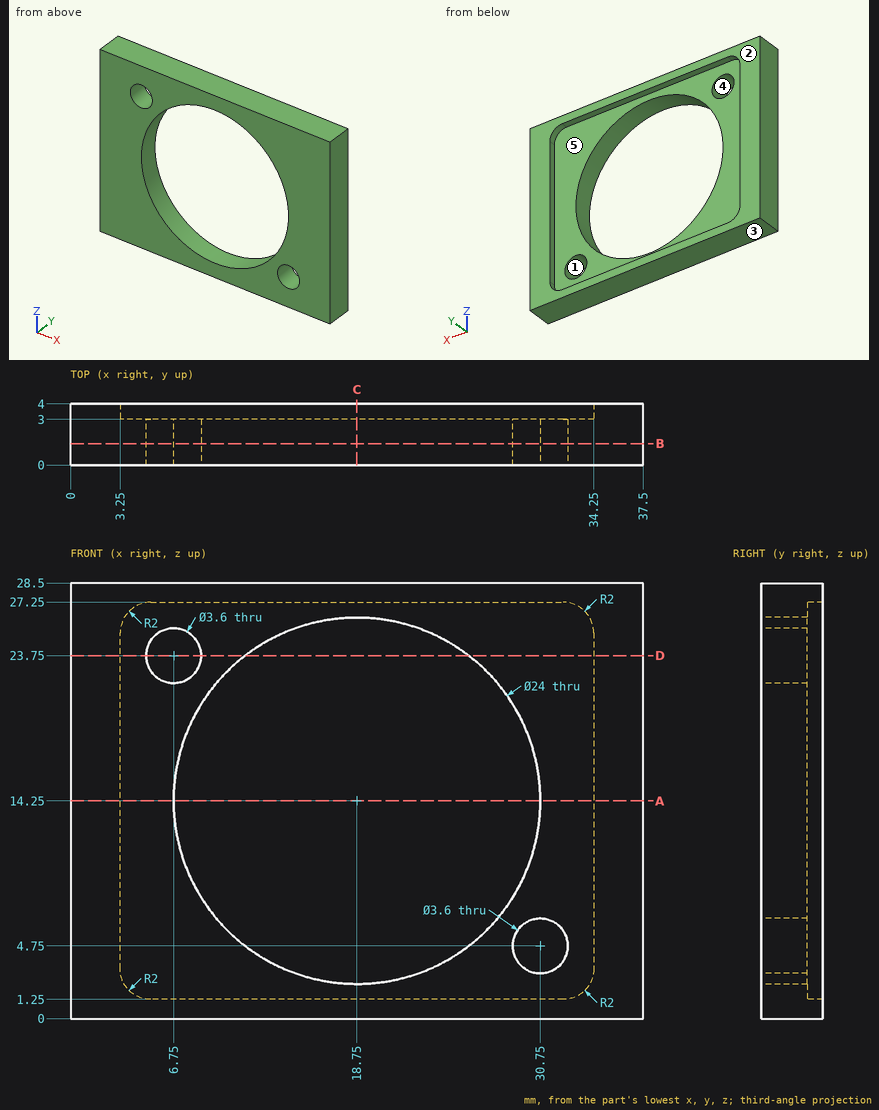
Check sheet for the drawn part. Datum: minimum x, y, z corner. Units: mm. A direction names the side the tool comes from. Give positions to 0.01 mm unless a question says otherwise; leave off trailing zeros. Loops run counter-clockwise (first coordinate to the right, second up) from the corner with the lowest first, then second, coordinate; pieces in that order, holes last. Notation, with made-up numbers: (17, 17) - (60, 17) arc R19 cw to (60, 46) - close; hole circle Ø3 at (-6, 11). An arc over 180 degrees is marked (long way). Write each question's results on one line, items separated by ' | '.
1) Mould release check, pull along Z, two halves, no side actions. Record for the marked faces 1, 2 and 3: pulls with the +Z half, pulls with the -Z half, needs draft (parallel to the pull), parting line crosses it, or undercut.
Solution:
face 1: undercut | face 2: needs draft | face 3: pulls with the -Z half
2) Depth check by flat-ended pin: P1, Ø4, axis at x = 6.75, z = 23.75, coming from the +Y side. Enter the tip coordinate at first touch or a pass-through.
Solution:
P1: y = 3
3) Sectioned sample at A-A on z = 14.25. Record the boundary of the cut face in (x, y), plus the area to 3 significant figures.
Solution:
outline: (0, 0) - (6.75, 0) - (6.75, 3) - (3.25, 3) - (3.25, 4) - (0, 4) - close; (30.75, 0) - (37.5, 0) - (37.5, 4) - (34.25, 4) - (34.25, 3) - (30.75, 3) - close | area: 47.0 mm2
4) Sectioned sample at B-B on y = 1.4. Record the boundary of the cut face in (x, z).
Solution:
outline: (0, 0) - (37.5, 0) - (37.5, 28.5) - (0, 28.5) - close; hole circle Ø3.6 at (6.75, 23.75); hole circle Ø24 at (18.75, 14.25); hole circle Ø3.6 at (30.75, 4.75)
5) Material ranges on L1, parallel to X at y = 1.45, z = 14.25; L2, parallel to Z at x = 27, y = 3.5; L3, parallel to X at y = 3.8, z = 17.75, recorded low to high. Write a range as from..to.
Solution:
L1: 0..6.75, 30.75..37.5 | L2: 0..1.25, 27.25..28.5 | L3: 0..3.25, 34.25..37.5
6) Sectioned sample at C-C on x = 18.75. Record the boundary of the cut face in (y, z), plus the area to 3 significant figures.
Solution:
outline: (0, 0) - (4, 0) - (4, 1.25) - (3, 1.25) - (3, 2.25) - (0, 2.25) - close; (0, 26.25) - (3, 26.25) - (3, 27.25) - (4, 27.25) - (4, 28.5) - (0, 28.5) - close | area: 16.0 mm2
7) Sectioned sample at D-D on z = 23.75. Record the boundary of the cut face in (x, y).
Solution:
outline: (0, 0) - (4.95, 0) - (4.95, 3) - (3.25, 3) - (3.25, 4) - (0, 4) - close; (8.55, 0) - (11.42, 0) - (11.42, 3) - (8.55, 3) - close; (26.08, 0) - (37.5, 0) - (37.5, 4) - (34.25, 4) - (34.25, 3) - (26.08, 3) - close
8) Tool access check on the marked faces 4 and 5. Record the directions out of +Z, -Z, +X, -X, +Y, -Y that give a thin tool (end or side, any length) a straight path to the whole face; none if there is none.
Solution:
face 4: +Y, -Y | face 5: +Y
